Solid Edge part; units mm, degrees
sketch "Sketch1" plane through (0, 0, 0) normal (0, 0, 1) x (1, 0, 0)
  circle A0 centre (0, 0) radius 1.27
extrude "Protrusion1" add sketch "Sketch1" along normal mid plane 38.1
sketch "Sketch2" plane through (0, 0, 0) normal (0, 0, 1) x (1, 0, 0)
  circle A0 centre (0, 0) radius 3.683
extrude "ExtrudedProtrusion_2" add sketch "Sketch2" along normal mid plane 28.575
sketch "Sketch3" plane through (0, 0, 0) normal (0, 0, 1) x (1, 0, 0)
  circle A0 centre (0, 0) radius 4.064
extrude "ExtrudedProtrusion_3" add sketch "Sketch3" along normal mid plane 25.4
Verification items for the finished model (mm, model axes). A direction names the side the tool comes from. Round coordinates to 2 decimals unless told otherwise and drop trailing zeros. Order: outer loops, then holes, each group sorted by start corner. A loop starts at its lowest first (then second) coordinate and runs counter-clockwise, first axis right, second up. Notation, with made-up numbers: (39.25, -9.5) -> (53.25, -9.5) arc R26 ccw to (53.25, 24.5) -> close; hole circle Ø9 at (63, -32). An arc over 180 degrees is marked (long way). Put each result on its own line as item: value.
1) Depth check by flat-ended pin: pin 1 (4 mm diameter, centred on x = -2.5, z = 3.5, fed in from -Y); pin 2 (1 mm diameter, centred on x = -1.5, z = 2.5, fed in from -Y); pin 3 (1.5 mm diameter, centred on x = -0.5, y = -2, fed in from +Z). Enter the tip coordinate at first touch or a pass-through.
Final values:
pin 1: stops at y = -4.03
pin 2: stops at y = -3.94
pin 3: stops at z = 14.29
2) Section check C-C (z = 4.5). Record the cut outline in (x, y), then the cut area to 3 significant figures.
Final values:
outline: circle Ø8.13 at (0, 0)
area: 51.9 mm^2
3) Section check A-A (x = 0). Record the cut outline in (y, z), then the cut area to 3 significant figures.
Final values:
outline: (-4.06, -12.7) -> (-3.68, -12.7) -> (-3.68, -14.29) -> (-1.27, -14.29) -> (-1.27, -19.05) -> (1.27, -19.05) -> (1.27, -14.29) -> (3.68, -14.29) -> (3.68, -12.7) -> (4.06, -12.7) -> (4.06, 12.7) -> (3.68, 12.7) -> (3.68, 14.29) -> (1.27, 14.29) -> (1.27, 19.05) -> (-1.27, 19.05) -> (-1.27, 14.29) -> (-3.68, 14.29) -> (-3.68, 12.7) -> (-4.06, 12.7) -> close
area: 254 mm^2
4) Section check D-D (x = 3.25). Record the cut outline in (y, z), then the cut area to 3 significant figures.
Final values:
outline: (-2.44, -12.7) -> (-1.73, -12.7) -> (-1.73, -14.29) -> (1.73, -14.29) -> (1.73, -12.7) -> (2.44, -12.7) -> (2.44, 12.7) -> (1.73, 12.7) -> (1.73, 14.29) -> (-1.73, 14.29) -> (-1.73, 12.7) -> (-2.44, 12.7) -> close
area: 135 mm^2
5) Material ranges on line 1 (X direction, y = -0.25, z = -8); line 2 (Z direction, x = -2.25, y = 3.25); line 3 (Z direction, x = -1.75, y = 1.25), recorded low to high.
Final values:
line 1: x = -4.06 to 4.06
line 2: z = -12.7 to 12.7
line 3: z = -14.29 to 14.29
6) Set-up check for faces 1 (the flat face through (0, 0, -19.05)), 2 (the cylindrical face through (1.699, -3.267, -13.483)), 3 (the cylindrical face through (-0.17, -1.26, 16.64)): record each of +Z, -Z, +X, -X, +Y, -Y from which the full face is reachable in a straight line by a thin tool's end or side.
Final values:
face 1: -Z, +X, -X, +Y, -Y
face 2: -Z
face 3: +Z
